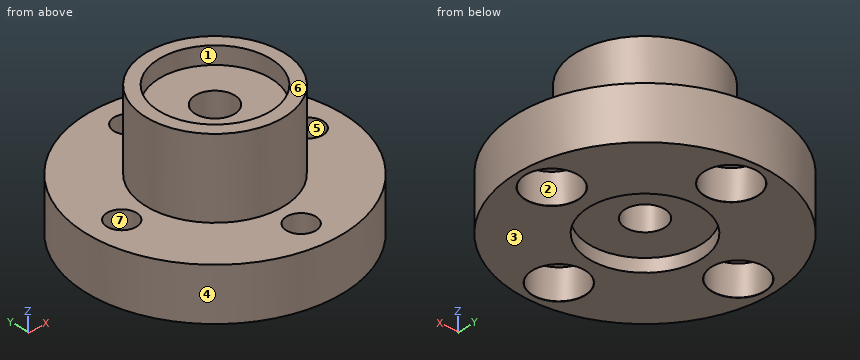
from build123d import *

# Parameters (mm, degrees)
SKETCH_1_R               = 19.5
EXTRUDE_1_DEPTH          = 8
SKETCH_2_R               = 10.5
EXTRUDE_2_DEPTH          = 12
SKETCH_3_R               = 3
CUT_EXTRUDE_1_DEPTH      = 35.066112194
SKETCH_4_R               = 8.5
CUT_EXTRUDE_3_DEPTH      = 2.65
CUT_EXTRUDE_START        = -2
SKETCH_5_R               = 8.5
CUT_EXTRUDE_4_DEPTH      = 2
PATTERN_CIRCULAR_1_COUNT = 4


with BuildPart() as part:
    # 草图1 → 凸台-拉伸1 (new body)
    with BuildSketch(Plane.XY):
        Circle(SKETCH_1_R)
    extrude(amount=EXTRUDE_1_DEPTH)

    # 草图2 → 凸台-拉伸2 (add)
    with BuildSketch(Plane.XY.offset(8)):
        Circle(SKETCH_2_R)
    extrude(amount=EXTRUDE_2_DEPTH)

    # 草图3 → 切除-拉伸1 (cut, through all)
    with BuildSketch(Plane(origin=(0, 0, 0), x_dir=(-1, 0, 0), z_dir=(0, 0, -1))):
        Circle(SKETCH_3_R)
    extrude(amount=-CUT_EXTRUDE_1_DEPTH, mode=Mode.SUBTRACT)

    # 草图4 → 切除-拉伸3 (cut)
    with BuildSketch(Plane.XY.offset(20)):
        Circle(SKETCH_4_R)
    extrude(amount=-CUT_EXTRUDE_3_DEPTH, mode=Mode.SUBTRACT)

    # 草图5 → 切除-拉伸4 (cut)
    with BuildSketch(Plane(origin=(0, 0, 0), x_dir=(-1, 0, 0), z_dir=(0, 0, -1)).offset(CUT_EXTRUDE_START)):
        with Locations(Location((0, 0, 0), (0, 0, 180))):
            Circle(SKETCH_5_R)
    extrude(amount=CUT_EXTRUDE_4_DEPTH, mode=Mode.SUBTRACT)

    # 草图7 → M4 六角圆柱头螺钉的柱形沉头孔1 (revolve, cut)
    with BuildSketch(Plane(origin=(0, 14.5, 0), x_dir=(0, 1, 0), z_dir=(1, 0, 0))):
        Polygon((0, 0), (0, 20), (2.25, 20), (2.25, 4.6), (4, 4.6), (4, 0.025), (4.025, 0), align=None)
    hole_wizard_m4_1 = revolve(axis=Axis((0, 14.5, -6.35), (0, 0, 1)), mode=Mode.SUBTRACT)

    # 阵列(圆周)1: M4 六角圆柱头螺钉的柱形沉头孔1 ×4 about axis
    pattern_circular_1_axis = Axis((0, 0, 0), (0, 0, 1))
    for i in range(1, PATTERN_CIRCULAR_1_COUNT):
        add(hole_wizard_m4_1.rotate(pattern_circular_1_axis, i * 360 / PATTERN_CIRCULAR_1_COUNT), mode=Mode.SUBTRACT)


solid = part.part
Source: CAD feature listing. Evaluate the final solid. Frame: model axes, mm. Face numbers are marked on the shaded views. A direction names the side the tool comes from. Round coordinates to 2 decimals unless told otherwise and drop trailing zeros. Loops run counter-clockwise (first coordinate to the right, second up) from the corner with the lowest first, then second, coordinate; pieces in that order, holes last.
Q1. Section D-D, the plane z = 10.5. Return loops of the section in (x, y).
Q2. Mould query, pull axis X, two halves, no side actions, for the marked faces 4, 5, 6 and 7. Classes: pulls with the +X half, pulls with the -X half, needs draft (parallel to the pull), parting line crosses it, or undercut.
Q3. Access query for the marked faces 1, 2 and 3. Directions: +Z, -Z, +X, -X, +Y, -Y. A direction counts if a zero-diameter tool reaches every point of the face in a straight line with its end or side. Return the directions, or none.
Q4. First-contact query: P1, Ø1, axis at x = -10.5, y = 15.5, coming from the +Z side; P2, Ø13.5, axis at x = 1, y = 1, coming from the +Z side; P3, Ø3.5, axis at x = 14.5, y = 0, coming from the +Z side; P4, Ø10, axis at x = 1.5, z = 11.5, coming from the +Y side. Flat tips, straight axial feed; report the tip coordinate or a pass-through.
Q5. Section A-A, the plane y = 14.5. Return loops of the section in (x, z) (3 decimals), plus the area to 3 significant figures.
Q6. Section B-B, the plane x = 0. State how many separate pieces and enclosed holes the cut face has, plus the area to 3 significant figures.
Q7. Ray query, line 1 (Y direction, x = 0, z = 17.9); line 2 (Z direction, x = -18, y = 5); line 3 (X direction, y = 0.5, z = 12.75). Return the intervals inside material, ascending.
Solutions:
1. outline: circle Ø21 at (0, 0); hole circle Ø6 at (0, 0)
2. face 4: parting line crosses it
2. face 5: undercut
2. face 6: needs draft
2. face 7: undercut
3. face 1: +Z
3. face 2: -Z
3. face 3: -Z, +X, -X, +Y, -Y
4. P1: stops at z = 8
4. P2: stops at z = 17.35
4. P3: passes through
4. P4: stops at y = 19.5
5. outline: (-13.038, 0) - (-4.025, 0) - (-4, 0.025) - (-4, 4.6) - (-2.25, 4.6) - (-2.25, 8) - (-13.038, 8) - close; (2.25, 4.6) - (4, 4.6) - (4, 0.025) - (4.025, 0) - (13.038, 0) - (13.038, 8) - (2.25, 8) - close
5. area: 157 mm2
6. separate pieces: 4
6. enclosed holes: 0
6. area: 289 mm2
7. line 1: y = -10.5 to -8.5, 8.5 to 10.5
7. line 2: z = 0 to 8
7. line 3: x = -10.49 to -2.96, 2.96 to 10.49
